Model file for the job. Use its own axes, mm. Face numbers are marked on the shaded views. A direction names the side the tool comes from. Coordinates: 2 decimals unless noted, no trailing zeros. Order: outer loops, then holes, each group sorted by start corner. A loop starts at its lowest first (then second) coordinate and runs counter-clockwise, first axis right, second up. Notation, with made-up numbers: (74, 3.5) -> (106, 3.5) arc R16 cw to (106, 10.5) -> close; hole circle Ø8 at (82, -12.5). An arc over 180 degrees is marked (long way). Write item = value, one per line. Start each with the question number.
Q1. Wall check: line 1 (Y direction, x = 0, z = 3.75); line 2 (X direction, y = 32, z = 1.25); line 3 (Y direction, x = 29.21, z = 2.75) (3 decimals). Give the ranges that are in metal, low to high. Write a range as from..to.
Q2. Cut at C-C, the plane x = 29.21. List the corners of the cut face in (y, z) (3 decimals), plus the area to 3 significant figures.
Q3. Cut at B-B, the plane x = -41. List the corners of the cut face in (y, z), plus the area to 3 significant figures.
Q4. Mould opens along Y. For the marked faces 4, 5, 6 and 7 say: +Y half, -Y half, draft (parallel to the pull), parting line (faces both ways), or undercut.
Q5. Cut at A-A, the plane y = -53. List the corners of the cut face in (x, z).
Q6. 3-axis set-ups, long thin cutter, end or side, ignore diameter. For the marked faces 1, 2 and 3: which of +Z, -Z, +X, -X, +Y, -Y reach the whole face in a straight line?
Q7. Flat gauge pins, fed straight in: pin 1 (3 mm diameter, centred on y = -26, z = 4.5, fed in from -X); pin 2 (2 mm diameter, centred on x = -42.5, y = 16, fed in from -Z); pin 3 (5 mm diameter, centred on x = -29.21, y = 3.81, fed in from +Z); pin 4 (1.5 mm diameter, centred on y = 14, z = 6.5, fed in from +X). Where does each tip first touch, or does it go through?
Q8. Cut at D-D, the plane z = 5.5. Give the number of separate pieces and of enclosed holes in the cut face, plus the area to 3 significant figures.
from build123d import *

# Parameters (mm, degrees)
F0_R     = 3.175
F0_R_2   = 10.5664
F1_DEPTH = 7.239


# Not quite as in the source:
# - a feature names something its author has since deleted; it is built from what else it names


with BuildPart() as f1:
    # F0 (on Top) → F1 (new body)
    with BuildSketch(Plane.XY):
        with BuildLine():
            ThreePointArc((49.499110543, 36.0206762632), (40.1908123412, 13.9051845012), (18.8098960555, 3.0150141596))
            ThreePointArc((18.8098960555, 3.0150141596), (18.9898791446, 1.5122797598), (19.05, 0))
            ThreePointArc((19.05, 0), (18.1264129292, -5.8596633283), (15.4452068954, -11.1511472037))
            ThreePointArc((15.4452068954, -11.1511472037), (38.9084897998, -15.0723597821), (62.437543059, -11.5673340383))
            ThreePointArc((62.437543059, -11.5673340383), (61.8751789356, 13.8326514264), (49.499110543, 36.0206762632))
        make_face()
        with Locations((29.21, -3.81)):
            Circle(F0_R, mode=Mode.SUBTRACT)
        with Locations((46.5836, 0)):
            Circle(F0_R_2, mode=Mode.SUBTRACT)
        with BuildLine():
            ThreePointArc((19.05, 0), (18.9898791446, 1.5122797598), (18.8098960555, 3.0150141596))
            ThreePointArc((18.8098960555, 3.0150141596), (16.2245432897, 9.9833208424), (11.1694758624, 15.4319573923))
            ThreePointArc((11.1694758624, 15.4319573923), (4.3764318058, 18.5404785442), (-3.0896344638, 18.7977833502))
            ThreePointArc((-3.0896344638, 18.7977833502), (-9.9628775585, 16.2371047528), (-15.3591721014, 11.2693536797))
            ThreePointArc((-15.3591721014, 11.2693536797), (-18.5170306594, 4.4746033968), (-18.8103206304, -3.0123641517))
            ThreePointArc((-18.8103206304, -3.0123641517), (-16.2548336089, -9.9339259281), (-11.2609801699, -15.3653124151))
            ThreePointArc((-11.2609801699, -15.3653124151), (-4.4663849388, -18.5190147032), (3.0188073829, -18.8092876522))
            ThreePointArc((3.0188073829, -18.8092876522), (9.994585264, -16.2176066483), (15.4452068954, -11.1511472037))
            ThreePointArc((15.4452068954, -11.1511472037), (18.1264129292, -5.8596633283), (19.05, 0))
        make_face()
        with BuildLine():
            ThreePointArc((-3.0490541894, 10.5671032828), (6.6115919208, 8.7890417858), (10.9982, 0))
            ThreePointArc((10.9982, 0), (8.7587082508, -6.6517240635), (2.9522592067, -10.5945537337))
            ThreePointArc((2.9522592067, -10.5945537337), (-5.4079074823, -9.5767917333), (-10.597009287, -2.9434329297))
            ThreePointArc((-10.597009287, -2.9434329297), (-9.601427461, 5.3640464159), (-3.0490541894, 10.5671032828))
        make_face(mode=Mode.SUBTRACT)
        with BuildLine():
            ThreePointArc((-3.0896344638, 18.7977833502), (4.3764318058, 18.5404785442), (11.1694758624, 15.4319573923))
            ThreePointArc((11.1694758624, 15.4319573923), (15.0487096917, 38.8348029597), (11.5431173905, 62.2965262207))
            ThreePointArc((11.5431173905, 62.2965262207), (-13.8155129183, 61.7441471546), (-35.9687104078, 49.3909655905))
            ThreePointArc((-35.9687104078, 49.3909655905), (-13.9597183633, 40.0799728948), (-3.0896344638, 18.7977833502))
        make_face()
        with Locations((0, 46.5836)):
            Circle(F0_R_2, mode=Mode.SUBTRACT)
        with Locations((3.81, 29.21)):
            Circle(F0_R, mode=Mode.SUBTRACT)
        with BuildLine():
            ThreePointArc((35.8851180212, -49.3004770417), (13.913777395, -40.0244664241), (3.0188073829, -18.8092876522))
            ThreePointArc((3.0188073829, -18.8092876522), (-4.4663849388, -18.5190147032), (-11.2609801699, -15.3653124151))
            ThreePointArc((-11.2609801699, -15.3653124151), (-15.1324011861, -38.7568750152), (-11.6267097771, -62.2060376719))
            ThreePointArc((-11.6267097771, -62.2060376719), (13.7319205316, -61.6536586058), (35.8851180212, -49.3004770417))
        make_face()
        with Locations((0, -46.5836)):
            Circle(F0_R_2, mode=Mode.SUBTRACT)
        with Locations((-3.81, -29.21)):
            Circle(F0_R, mode=Mode.SUBTRACT)
        with BuildLine():
            ThreePointArc((-18.8103206304, -3.0123641517), (-18.5170306594, 4.4746033968), (-15.3591721014, 11.2693536797))
            ThreePointArc((-15.3591721014, 11.2693536797), (-38.7496809324, 15.1400454081), (-62.1976706421, 11.6343448498))
            ThreePointArc((-62.1976706421, 11.6343448498), (-61.6452915761, -13.7242854589), (-49.292110012, -35.8774829485))
            ThreePointArc((-49.292110012, -35.8774829485), (-40.0193213234, -13.909615697), (-18.8103206304, -3.0123641517))
        make_face()
        with Locations((-46.5836, 0)):
            Circle(F0_R_2, mode=Mode.SUBTRACT)
        with Locations((-29.21, 3.81)):
            Circle(F0_R, mode=Mode.SUBTRACT)
    extrude(amount=F1_DEPTH)


solid = f1.part
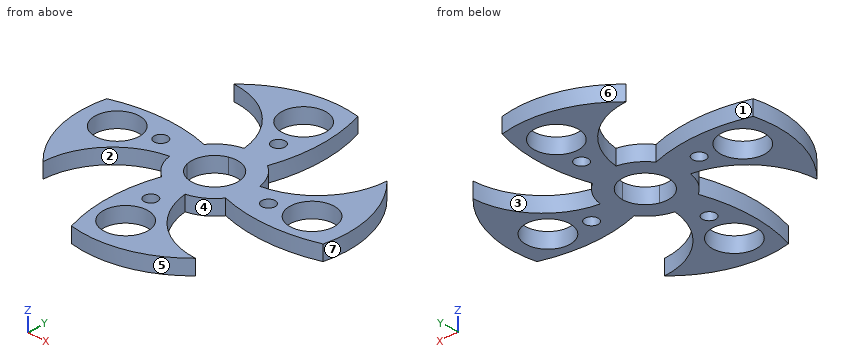
Here are the results:
q1.line_1 = -63.49..-57.15, -36.02..-11, 11..36.02, 57.15..63.58
q1.line_2 = -7.52..2.29, 5.33..14.69, 49.07..52.9
q1.line_3 = -54.6..-48.307, -14.366..-6.985, -0.635..5.958
q2.outline = (-54.6, 0) -> (-48.307, 0) -> (-48.307, 7.239) -> (-54.6, 7.239) -> close; (-14.366, 0) -> (-6.985, 0) -> (-6.985, 7.239) -> (-14.366, 7.239) -> close; (-0.635, 0) -> (5.958, 0) -> (5.958, 7.239) -> (-0.635, 7.239) -> close
q2.area = 147 mm²
q3.outline = (-15.01, 0) -> (-8.97, 0) -> (-8.97, 7.24) -> (-15.01, 7.24) -> close; (8.97, 0) -> (15.12, 0) -> (15.12, 7.24) -> (8.97, 7.24) -> close
q3.area = 88.3 mm²
q4.face_4 = undercut
q4.face_5 = -Y half
q4.face_6 = +Y half
q4.face_7 = parting line
q5.outline = (-13.9, 0) -> (-8.4, 0) -> (-8.4, 7.24) -> (-13.9, 7.24) -> close; (8.4, 0) -> (31.47, 0) -> (31.47, 7.24) -> (8.4, 7.24) -> close
q6.face_1 = +Z, -Z
q6.face_2 = +Z, -Z, -Y
q6.face_3 = +Z, -Z, +Y
q7.pin_1 = -57.4
q7.pin_2 = 0
q7.pin_3 = through
q7.pin_4 = 62.03
q8.separate_pieces = 1
q8.enclosed_holes = 9
q8.area = 4,540 mm²
